For this review, use the dimensioned drawing (mm, ordinates from the lowest corner) and the shaded views. A direction names the side the tool comes from. Coordinates: 2 decimals unless noted, no trailing zeros. Write each loop counter-clockwise with the first axis right and the second up, starting at its lowest first coordinate (ties: lowest second). Pieces come first, ordered by that corner, then holes.
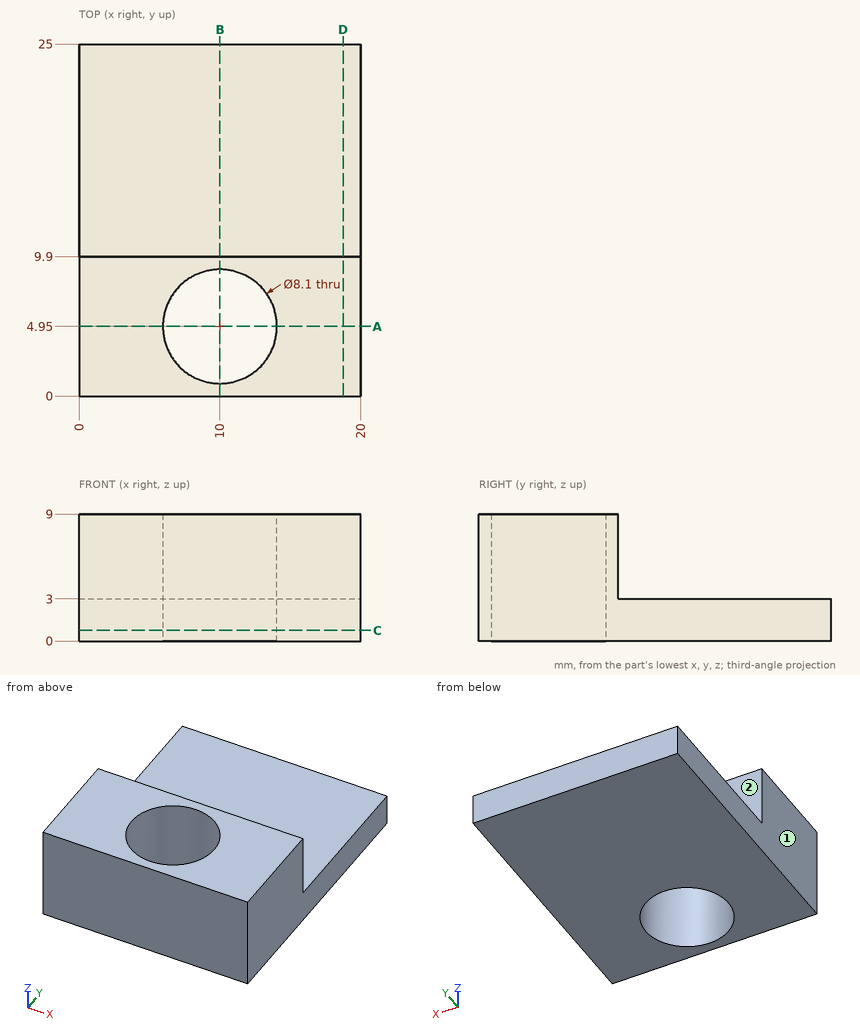
Item 1: For pin 1 (1.8 mm diameter, centred on x = 7.5, z = 6, fed in from +Y); pin 2 (1.5 mm diameter, centred on y = 6.5, z = 3.5, fed in from -X); pin 3 (4.5 mm diameter, centred on x = 8.5, y = 14.5, fed in from +Z), all flat-tipped, find the tip position at first contact; note any pin that passes through.
Solved:
pin 1: stops at y = 9.9
pin 2: stops at x = 0
pin 3: stops at z = 3
Item 2: To check wall thickness, follow line 1 along Y through (x, z) = (10, 4); line 2 along Z through (x, y) = (16.5, 17.5); line 3 along Y through (x, z) = (14.5, 8.5). State the ranges of each line that lie inside material, in increasing order.
Solved:
line 1: y = 0 to 0.9, 9 to 9.9
line 2: z = 0 to 3
line 3: y = 0 to 9.9
Item 3: Take a section at D-D, the plane x = 18.75. Write out the cut boundary in (y, z).
Solved:
outline: (0, 0) - (25, 0) - (25, 3) - (9.9, 3) - (9.9, 9) - (0, 9) - close
Item 4: Take a section at C-C, the plane z = 0.75. Write out the cut boundary in (x, y).
Solved:
outline: (0, 0) - (20, 0) - (20, 25) - (0, 25) - close; hole circle Ø8.1 at (10, 4.95)
Item 5: Take a section at A-A, the plane y = 4.95. Write out the cut boundary in (x, z).
Solved:
outline: (0, 0) - (5.95, 0) - (5.95, 9) - (0, 9) - close; (14.05, 0) - (20, 0) - (20, 9) - (14.05, 9) - close
Item 6: Machinability: for the marked faces 1 and 2, which of the approach directions +Z, -Z, +X, -X, +Y, -Y give a long, thin tool a straight path to every point of the face, cutting with its end or side? Answer none if there is none.
Solved:
face 1: +Z, -Z, -X, +Y, -Y
face 2: +Z, +X, -X, +Y
Item 7: Take a section at B-B, the plane x = 10. Write out the cut boundary in (y, z), plus the area to 3 significant figures.
Solved:
outline: (0, 0) - (0.9, 0) - (0.9, 9) - (0, 9) - close; (9, 0) - (25, 0) - (25, 3) - (9.9, 3) - (9.9, 9) - (9, 9) - close
area: 61.5 mm2
